from build123d import *

# Parameters (mm, degrees)
ESBO_O1_W                = 200
ESBO_O1_H                = 200
RESSALTO_EXTRUS_O2_DEPTH = 200
ESBO_O4_W                = 91.052715104
ESBO_O4_H                = 180
ESBO_O4_W_2              = 83.947284896
ESBO_O4_H_2              = 68.664679647
ESBO_O4_H_3              = 106.335320353
CORTE_EXTRUS_O2_DEPTH    = 190
FILETE2_R                = 7
FILETE3_R                = 7
FILETE4_R                = 7
FILETE5_R                = 7
FILETE6_R                = 7
ESBO_O5_R                = 5
CORTE_EXTRUS_O3_DEPTH    = 10
ESBO_O6_R                = 10
CORTE_EXTRUS_O4_DEPTH    = 10


with BuildPart() as part:
    # Esboço1 → Ressalto-extrusão2 (new body)
    with BuildSketch(Plane.XY):
        with Locations((100, 100)):
            Rectangle(ESBO_O1_W, ESBO_O1_H)
    extrude(amount=RESSALTO_EXTRUS_O2_DEPTH)

    # Esboço4 → Corte-extrusão2 (cut)
    with BuildSketch(Plane(origin=(0, 0, 0), x_dir=(-1, 0, 0), z_dir=(0, 0, -1))):
        with Locations((-144.473642448, 100)):
            Rectangle(ESBO_O4_W, ESBO_O4_H)
        with Locations((-51.973642448, 44.332339823)):
            Rectangle(ESBO_O4_W_2, ESBO_O4_H_2)
        with Locations((-51.973642448, 136.832339824)):
            Rectangle(ESBO_O4_W_2, ESBO_O4_H_3)
    extrude(amount=-CORTE_EXTRUS_O2_DEPTH, mode=Mode.SUBTRACT)

    # Filete2
    filete2_edges = [part.edges().sort_by_distance(p)[0] for p in [
        (0, 0, 100),
        (0, 200, 100),
        (200, 200, 100),
        (200, 0, 100),
    ]]
    fillet(filete2_edges, radius=FILETE2_R)

    # Filete3
    filete3_edges = [part.edges().sort_by_distance(p)[0] for p in [
        (190, 10, 95),
        (190, 190, 95),
        (98.947284896, 190, 95),
        (98.947284896, 10, 95),
        (93.947284896, 10, 95),
        (93.947284896, 78.664679647, 95),
        (10, 78.664679647, 95),
        (10, 10, 95),
        (10, 190, 95),
        (10, 83.664679647, 95),
    ]]
    fillet(filete3_edges, radius=FILETE3_R)

    # Filete4
    filete4_edges = [part.edges().sort_by_distance(p)[0] for p in [
        (12.050252532, 187.949747468, 190),
        (12.050252532, 85.714932179, 190),
        (93.947284896, 136.832339824, 190),
        (55.473642448, 83.664679647, 190),
        (93.947284896, 44.332339824, 190),
        (51.973642448, 78.664679647, 190),
        (51.973642448, 10, 190),
        (10, 44.332339824, 190),
        (12.050252532, 12.050252532, 190),
        (12.050252532, 76.614427115, 190),
        (91.897032365, 12.050252532, 190),
        (91.897032365, 76.614427115, 190),
        (190, 100, 190),
        (144.473642448, 190, 190),
        (144.473642448, 10, 190),
        (98.947284896, 100, 190),
        (100.997537428, 187.949747468, 190),
        (100.997537428, 12.050252532, 190),
        (187.949747468, 12.050252532, 190),
        (187.949747468, 187.949747468, 190),
        (10, 136.832339824, 190),
        (55.473642448, 190, 190),
    ]]
    fillet(filete4_edges, radius=FILETE4_R)

    # Filete5
    filete5_edges = [part.edges().sort_by_distance(p)[0] for p in [
        (0, 100, 200),
        (100, 200, 200),
        (100, 0, 200),
        (200, 100, 200),
        (197.949747468, 2.050252532, 200),
        (2.050252532, 2.050252532, 200),
        (197.949747468, 197.949747468, 200),
        (2.050252532, 197.949747468, 200),
    ]]
    fillet(filete5_edges, radius=FILETE5_R)

    # Filete6
    # the kernel refuses this fillet: 7 mm, written as the material it adds along each edge
    with BuildSketch(Plane(origin=(86.947284896, 183, 183), x_dir=(1, 0, 0), z_dir=(0, 1, 0))) as filete6_piece_1_section:
        Polygon((0, 0), (FILETE6_R * 1.02, 0), (FILETE6_R * 1.02, -FILETE6_R * 1.02), (0, -FILETE6_R * 1.02), align=None)
    filete6_piece_1 = extrude(amount=FILETE6_R * 1.02, mode=Mode.PRIVATE)
    filete6_piece_1 = filete6_piece_1 - Plane(origin=(86.947284896, 183, 183), x_dir=(-0.7071067811865475, 0, -0.7071067811865475), z_dir=(0, 1, 0)) * Sphere(FILETE6_R, mode=Mode.PRIVATE)
    add(filete6_piece_1)
    with BuildSketch(Plane(origin=(86.947284896, 90.664679647, 183), x_dir=(0, -1, 0), z_dir=(1, 0, 0))) as filete6_piece_2_section:
        Polygon((0, 0), (FILETE6_R * 1.02, 0), (FILETE6_R * 1.02, -FILETE6_R * 1.02), (0, -FILETE6_R * 1.02), align=None)
    filete6_piece_2 = extrude(amount=FILETE6_R * 1.02, mode=Mode.PRIVATE)
    filete6_piece_2 = filete6_piece_2 - Plane(origin=(86.947284896, 90.664679647, 183), x_dir=(0, 0.7071067811865475, -0.7071067811865475), z_dir=(1, 0, 0)) * Sphere(FILETE6_R, mode=Mode.PRIVATE)
    add(filete6_piece_2)
    with BuildSketch(Plane(origin=(93.947284896, 83.664679647, 0), x_dir=(0, 1, 0), z_dir=(0, 0, 1)), Plane(origin=(93.947284896, 190, 0), x_dir=(-1, 0, 0), z_dir=(0, 0, 1))) as filete6_piece_3:
        with BuildLine():
            CenterArc((FILETE6_R, FILETE6_R), FILETE6_R, 180, 90)
            Line((0, FILETE6_R), (0, 0))
            Line((0, 0), (FILETE6_R, 0))
        make_face()
    extrude(amount=183)

    # Esboço5 → Corte-extrusão3 (cut)
    with BuildSketch(Plane(origin=(0, 83.664679647, 0), x_dir=(1, 0, 0), z_dir=(0, 1, 0))):
        with Locations(Location((53.753482912, -10, 0), (0, 0, 270))):
            Circle(ESBO_O5_R)
    extrude(amount=-CORTE_EXTRUS_O3_DEPTH, mode=Mode.SUBTRACT)

    # Esboço6 → Corte-extrusão4 (cut)
    with BuildSketch(Plane.ZY):
        with Locations((173, 172.46544245)):
            Circle(ESBO_O6_R)
    extrude(amount=-CORTE_EXTRUS_O4_DEPTH, mode=Mode.SUBTRACT)


solid = part.part
The model under review builds one solid part; all positions refer to its coordinate system, in mm. A direction names the side the tool comes from. Coordinates: 2 decimals unless noted, no trailing zeros. Write each loop counter-clockwise with the first axis right and the second up, starting at its lowest first coordinate (ties: lowest second). Pieces come first, ordered by that corner, then holes. Notation, with made-up numbers: (81.25, -12.75) - (89.25, -12.75) arc R16 ccw to (89.25, 14.25) - close; hole circle Ø4 at (34.5, 6.5). An arc over 180 degrees is marked (long way). Answer as CSV lines item,"result".
(1) We need section B-B (x = 69). Give the boundary of the cut face in (y, z).
Data:
outline,"(0, 0) - (10, 0) - (10, 183) arc R7 cw to (17, 190) - (71.66, 190) arc R7 cw to (78.66, 183) - (78.66, 0) - (83.66, 0) - (83.66, 183) arc R7 cw to (90.66, 190) - (183, 190) arc R7 cw to (190, 183) - (190, 0) - (200, 0) - (200, 193) arc R7 ccw to (193, 200) - (7, 200) arc R7 ccw to (0, 193) - close"
(2) We need section C-C (y = 111). Give the boundary of the cut face in (x, z).
Data:
outline,"(0, 0) - (10, 0) - (10, 183) arc R7 cw to (17, 190) - (86.95, 190) arc R7 cw to (93.95, 183) - (93.95, 0) - (98.95, 0) - (98.95, 183) arc R7 cw to (105.95, 190) - (183, 190) arc R7 cw to (190, 183) - (190, 0) - (200, 0) - (200, 193) arc R7 ccw to (193, 200) - (7, 200) arc R7 ccw to (0, 193) - close"
(3) Mouldability with a two-part tool opening along Y and no side actions: class faces 3 (the cylindrical face through (197.9, 2, 97.9)), 4 (the cylindrical face through (143.9, 188, 187.9)), 5 (the cylindrical face through (197.9, 198, 97.9)) as pulls with the +Y half, pulls with the -Y half, needs draft (parallel to the pull), parting line crosses it, or undercut.
Data:
face 3,"pulls with the -Y half"
face 4,"undercut"
face 5,"pulls with the +Y half"
(4) Tool access review of faces 1 (the cylindrical face through (2, 101.3, 197.9)), 2 (the cylindrical face through (51.484, 76.669, 187.895)): name each direction out of +Z, -Z, +X, -X, +Y, -Y from which nothing blocks a thin tool from reaching the whole face with its end or side.
Data:
face 1,"+Z, -X, +Y, -Y"
face 2,"-Z"
(5) For line 1 along Y through (x, z) = (33, 123); line 2 along X through (y, z) = (81, 10); line 3 along X through (y, z) = (132.5, 30), list the stretches that pass through material, from the lowest coordinate up. Write a range as [from, to].
Data:
line 1,"y = [0, 10], [78.66, 83.66], [190, 200]"
line 2,"x = [0, 48.75], [58.75, 98.95], [190, 200]"
line 3,"x = [0, 10], [93.95, 98.95], [190, 200]"
(6) Clearance check with a flat-ended pin moving along its axis: pin 1 Ø1 at (x, y) = (176.5, 170.5) entering from -Z. State where the tip first meets the part, or that it passes through.
Data:
pin 1,"stops at z = 190"
(7) We need section A-A (z = 144.5). Count the separate pieces of the cut face and the enclosed holes in it, plus the area to 3 significant figures.
Data:
separate pieces,"1"
enclosed holes,"3"
area,"9,000 mm2"
